from build123d import *

# Parameters (mm, degrees)
CROQUIS1_R              = 9
CROQUIS1_R_2            = 1.5
SALIENTE_EXTRUIR1_DEPTH = 4
CORTAR_EXTRUIR1_DEPTH   = 15
CORTAR_EXTRUIR2_DEPTH   = 10


with BuildPart() as part:
    # Croquis1 → Saliente-Extruir1 (new body)
    with BuildSketch(Plane.XY):
        Circle(CROQUIS1_R)
        Circle(CROQUIS1_R_2, mode=Mode.SUBTRACT)
    extrude(amount=SALIENTE_EXTRUIR1_DEPTH)

    # Croquis2 → Cortar-Extruir1 (cut)
    with BuildSketch(Plane(origin=(0, 0, 0), x_dir=(0, 0, -1), z_dir=(1, 0, 0))):
        Polygon((-1.5, -5.6), (-4, 0), (-4, -9), (-1.5, -9), align=None)
    extrude(amount=-CORTAR_EXTRUIR1_DEPTH, mode=Mode.SUBTRACT)

    # Croquis3 → Cortar-Extruir2 (cut)
    with BuildSketch(Plane(origin=(0, 0, 0), x_dir=(1, 0, 0), z_dir=(0, 1, 0))):
        Polygon((0, -1.5), (0, -4), (4.803477962, -4), (0.798212, -1.5), align=None)
    extrude(amount=-CORTAR_EXTRUIR2_DEPTH, mode=Mode.SUBTRACT)


solid = part.part
CAD build for the part. Positions are in the model's coordinates, mm. A direction names the side the tool comes from. Round coordinates to 2 decimals unless told otherwise and drop trailing zeros. Write each loop counter-clockwise with the first axis right and the second up, starting at its lowest first coordinate (ties: lowest second). Pieces come first, ordered by that corner, then holes.
(1) 3-axis set-ups, long thin cutter, end or side, ignore diameter. For faces 5 (the face through (-1.11, 1.01, 1.97)), 6 (the face through (2.83, -4.42, 2.77)): which of +Z, -Z, +X, -X, +Y, -Y reach the whole face in a straight line?
(2) Slice it at C-C, the plane x = -4.75. Write the cut outline in (y, z), and give its area (3 significant figures).
(3) Slice it at B-B, the plane y = -1.75. Write the cut outline in (x, z).
(4) Slice it at A-A, the plane z = 0.6. Write the cut outline in (x, y).
(5) Drop flat-ended pins along their axis: P1, Ø2.5, axis at x = -4, y = -5.5, coming from the +Z side; P2, Ø2, axis at y = 5.5, z = 1, coming from the +X side; P3, Ø1.5, axis at x = 0, z = 2.5, coming from the -Y side. Give the stop position or say it passes through.
(6) Mould opens along X. For faces 1 (the face through (0, -3, 2)), 2 (the face through (4.84, 7.59, 1.97)), 3 (the face through (-4.44, -2.84, 2.73)), 4 (the face through (2, 0, 3)) say: pulls with the +X half, pulls with the -X half, needs draft (parallel to the pull), parting line crosses it, or undercut.
(7) Slice it at D-D, the plane z = 3.1. Write the cut outline in (x, y), and give its area (3 significant figures).
(8) Probe line 1 along Y through (x, z) = (0, 1); line 2 along X through (y, z) = (-3, 1.95); line 3 along Y through (x, z) = (-0.25, 2.2). List the from-to ranges inside material, lowest first.
From the geometry:
1. face 5: +Z, -Z
1. face 6: +Z, -Y
2. outline: (-7.64, 0) - (7.64, 0) - (7.64, 4) - (0, 4) - (-5.6, 1.5) - (-7.64, 1.5) - close
2. area: 49.0 mm2
3. outline: (-8.83, 0) - (8.83, 0) - (8.83, 4) - (4.8, 4) - (0.8, 1.5) - (0, 1.5) - (0, 3.22) - (-8.83, 3.22) - close
4. outline: circle Ø18 at (0, 0); hole circle Ø3 at (0, 0)
5. P1: stops at z = 2.1
5. P2: stops at x = 7.79
5. P3: stops at y = -5.04
6. face 1: undercut
6. face 2: parting line crosses it
6. face 3: needs draft
6. face 4: undercut
7. outline: (-8.77, -2.02) - (0, -2.02) - (0, -1.5) arc R1.5 cw (long way) to (1.5, 0) - (3.36, 0) - (3.36, -8.35) arc R9 ccw (long way) to start
7. area: 174 mm2
8. line 1: y = -9 to -1.5, 1.5 to 9
8. line 2: x = -8.49 to 0, 1.52 to 8.49
8. line 3: y = -4.03 to -1.48, 1.48 to 9
